CAD build for the part. Positions are in the model's coordinates, mm. A direction names the side the tool comes from. Give positions to 0.01 mm unless a question says otherwise; leave off trailing zeros. Loops run counter-clockwise (first coordinate to the right, second up) from the corner with the lowest first, then second, coordinate; pieces in that order, holes last. Notation, with made-up numbers: M -34,-37 L 2,-37 A13 cw 2,-19 Z; hole C -14,76.5 d2. An arc over 180 degrees is marked long. One line per question, with ' | ' between items.
```python
from build123d import *

# Parameters (mm, degrees)
EXTRUS_O1_DEPTH               = 14
EXTRUS_O2_REACH               = 52.629
ESBO_O2_R                     = 2.5
FURO_ROSCADO_DE_M4X0_71_D     = 3.3
FURO_ROSCADO_DE_M4X0_71_DEPTH = 11.5
FURO_ROSCADO_DE_M4X0_71_TIP   = 0.991420021
ESBO_O5_R                     = 2.75
EXTRUS_O3_DEPTH               = 55.334611437
ESBO_O6_R                     = 3.5
EXTRUS_O4_DEPTH               = 3


with BuildPart() as part:
    # Esboço1 → Extrusão1 (new body)
    with BuildSketch(Plane.XY):
        with BuildLine():
            Line((0, 0), (0, 42))
            Line((0, 42), (-6, 42))
            Line((-6, 42), (-6, 31))
            Line((-6, 31), (-37.5, 31))
            Line((-37.5, 31), (-37.5, 21.75))
            Line((-37.5, 21.75), (-28.95294045, 21.75))
            ThreePointArc((-28.95294045, 21.75), (-17, 21), (-28.95294045, 20.25))
            Line((-28.95294045, 20.25), (-37.5, 20.25))
            Line((-37.5, 20.25), (-37.5, 11))
            Line((-37.5, 11), (-6, 11))
            Line((-6, 11), (-6, 0))
            Line((-6, 0), (0, 0))
        make_face()
    extrude(amount=EXTRUS_O1_DEPTH)

    # Esboço2 → Extrusão2 (cut, up to next)
    with BuildSketch(Plane(origin=(0, 31, 0), x_dir=(1, 0, 0), z_dir=(0, 1, 0)), mode=Mode.PRIVATE) as extrus_o2_sk1:
        with Locations(Location((-33.25, -7, 0), (0, 0, 270))):
            Circle(ESBO_O2_R)
    extrus_o2_tool1 = extrude(extrus_o2_sk1.sketch, amount=-EXTRUS_O2_REACH, mode=Mode.PRIVATE) & part.part
    add(extrus_o2_tool1.solids().sort_by_distance((-33.25, 31, 7))[0], mode=Mode.SUBTRACT)

    # Furo roscado de M4x0.71
    with Locations(Plane(origin=(-33.25, 20.25, 7), x_dir=(0, 0, 1), z_dir=(0, 1, 0))):
        with Locations((0, 0)):
            Hole(FURO_ROSCADO_DE_M4X0_71_D / 2, depth=FURO_ROSCADO_DE_M4X0_71_DEPTH)
            with Locations((0, 0, -(FURO_ROSCADO_DE_M4X0_71_DEPTH + FURO_ROSCADO_DE_M4X0_71_TIP / 2))):  # 118° drill point
                Cone(0, FURO_ROSCADO_DE_M4X0_71_D / 2, FURO_ROSCADO_DE_M4X0_71_TIP, mode=Mode.SUBTRACT)

    # Esboço5 → Extrusão3 (cut, through all)
    with BuildSketch(Plane.ZY.offset(6)):
        with Locations(Location((7, 37, 0), (0, 0, 270))):
            Circle(ESBO_O5_R)
        with Locations(Location((7, 5, 0), (0, 0, 270))):
            Circle(ESBO_O5_R)
    extrude(amount=-EXTRUS_O3_DEPTH, mode=Mode.SUBTRACT)

    # Esboço6 → Extrusão4 (cut)
    with BuildSketch(Plane(origin=(0, 31, 0), x_dir=(1, 0, 0), z_dir=(0, 1, 0))):
        with Locations(Location((-33.25, -7, 0), (0, 0, 270))):
            Circle(ESBO_O6_R)
    extrude(amount=-EXTRUS_O4_DEPTH, mode=Mode.SUBTRACT)


solid = part.part
```
Item 1: 3-axis set-ups, long thin cutter, end or side, ignore diameter. For faces 4 (the flat face through (-22, 11, 7)), 5 (the flat face through (-6, 34, 7)), 6 (the flat face through (-35, 21.75, 5)), 7 (the cylindrical face through (-29.78, 29.52, 6.54)): which of +Z, -Z, +X, -X, +Y, -Y reach the whole face in a straight line?
Conclusion:
face 4: +Z, -Z, -X, -Y | face 5: +Z, -Z, -X, +Y | face 6: +Z, -Z, -X | face 7: +Y
Item 2: Mould opens along Z. For faces 1 (the flat face through (0, 21, 7)), 2 (the flat face through (-15, 21, 0)), 3 (the flat face through (-35, 28, 9)) say: pulls with the +Z half, pulls with the -Z half, needs draft (parallel to the pull), parting line crosses it, or undercut.
Conclusion:
face 1: needs draft | face 2: pulls with the -Z half | face 3: undercut
Item 3: Drill centre lines: line 1 along Y through (x, z) = (-32.5, 11.5); line 2 along Z through (x, y) = (-4.7, 5); line 3 along X through (y, z) = (23.5, 7). Where is each one in solid material? Low to high. Write a range as [from, to].
Conclusion:
line 1: [11, 20.25], [21.75, 31] | line 2: [0, 4.25], [9.75, 14] | line 3: [-37.5, -35.75], [-30.75, -28.45], [-17.55, 0]
Item 4: Saw through at B-B on x = -33.25. Give the cut face in (y, z).
Conclusion:
outline: M 11,0 L 20.25,0 L 20.25,5.35 L 11,5.35 Z; M 11,8.65 L 20.25,8.65 L 20.25,14 L 11,14 Z; M 21.75,0 L 31,0 L 31,3.5 L 28,3.5 L 28,4.5 L 21.75,4.5 Z; M 21.75,9.5 L 28,9.5 L 28,10.5 L 31,10.5 L 31,14 L 21.75,14 Z
Item 5: Saw through at C-C on y = 5. Give the cut face in (x, z).
Conclusion:
outline: M -6,0 L 0,0 L 0,4.25 L -6,4.25 Z; M -6,9.75 L 0,9.75 L 0,14 L -6,14 Z
Item 6: Drop flat-ended pins along their axis: P1, Ø5.5, axis at y = 8, z = 4, coming from the -X side; P2, Ø7, axis at y = 5, z = 7, coming from the +X side; P3, Ø4, axis at x = -33.25, z = 7, coming from the -Y side; P4, Ø5, axis at x = -18.5, z = 7, coming from the +Y side. Give the stop position or say it passes through.
Conclusion:
P1: x = -6 | P2: x = 0 | P3: y = 11 | P4: y = 31
Item 7: Saw through at A-A on z = 7. State how many separate pieces and enclosed holes the cut face has, and give its area (3 significant figures).
Conclusion:
separate pieces: 5 | enclosed holes: 0 | area: 607 mm²
Item 8: Saw through at D-D on x = -23. Give the cut face in (y, z), and give its area (3 significant figures).
Conclusion:
outline: M 11,0 L 15,0 L 15,14 L 11,14 Z; M 27,0 L 31,0 L 31,14 L 27,14 Z | area: 112 mm²
